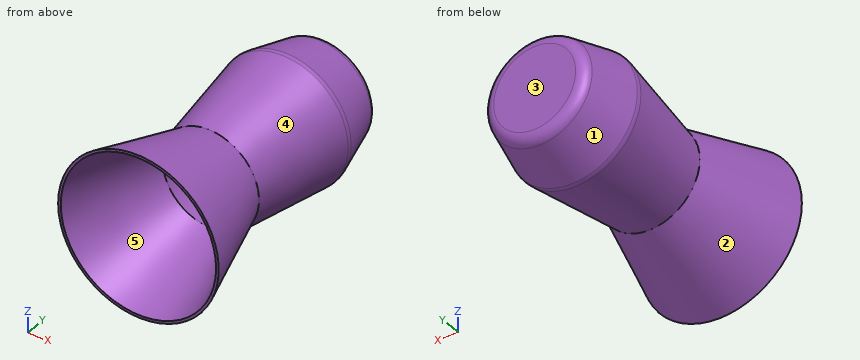
Autodesk Fusion 360 part; units mm, degrees
sketch "Esquisse1" plane through (0, 0, 0) normal (0, 0, 1) x (1, 0, 0)
  line L0 (0, 0) -> (-65, 0)
  line L1 (-65, 0) -> (-40, 80)
  line L2 (-40, 80) -> (-52.5, 165)
  line L3 (-52.5, 165) -> (-40, 210)
  line L4 (-40, 210) -> (0, 210)
  line L5 (0, 210) -> (0, 0)
  dimension "d1" = 65
  dimension "d3" = 45
  dimension "d4" = 85
  dimension "d5" = 80
  dimension "d6" = 40
  dimension "d7" = 52.5
  dimension "d8" = 40
revolve "Révolution1" add sketch "Esquisse1" angle 360 about axis through (0, 210, 0) along (0, -1, 0)
fillet "Congé1" radius 9 1 edges at (-48.9472, 165, 18.9848)
fillet "Congé2" radius 9 1 edges at (-37.2931, 210, 14.4646)
shell "Coque1" thickness 2 removed faces 1 at (20.2416, 0, -0.2148)
The model under review builds one solid part; all positions refer to its coordinate system, in mm. Face numbers are marked on the shaded views. A direction names the side the tool comes from. Round coordinates to 2 decimals unless told otherwise and drop trailing zeros. Order: outer loops, then holes, each group sorted by start corner. A loop starts at its lowest first (then second) coordinate and runs counter-clockwise, first axis right, second up. Notation, with made-up numbers: (78.25, 58) -> (124.25, 58) arc R20 ccw to (124.25, 88) -> close; hole circle Ø11 at (-5, 35.5). An arc over 180 degrees is marked (long way). One line per item, written item: value. Start each with the question number.
Q1. Clearance check with flat-ended pins moving along their axes: pin 1 Ø10 at (y, z) = (47, 43.5) entering from -X; pin 2 Ø8 at (y, z) = (167.5, -20.5) entering from -X; pin 3 Ø20 at (x, z) = (13, -3.5) entering from -Y. State where each tip first meets the part, or that it passes through.
Q2. Mouldability with a two-part tool opening along X and no side actions: class the marked faces 3, 4 and 5 as released by +X, released by -X, zero draft, split by the parting line, or undercut.
Q3. Machinability: for the marked faces 1 and 2, which of the approach directions +Z, -Z, +X, -X, +Y, -Y give a long, thin tool a straight path to every point of the face, cutting with its end or side? Answer none if there is none.
Q4. Take a section at A-A (y = 25). Write out the cut boundary in (x, z) (1 decimal), and give its area (3 significant figures).
Q5. Wall thickness on line 1 (Z direction, x = 10.5, y = 60); line 2 (X direction, y = 92, z = -15); line 3 (X direction, y = 52.5, z = 35): over which ranges is each line inside the solid? List them lowest first.
Reported:
1. pin 1: stops at x = -32.87
1. pin 2: stops at x = -49.41
1. pin 3: stops at y = 208
2. face 3: zero draft
2. face 4: split by the parting line
2. face 5: undercut
3. face 1: +Y
3. face 2: none
4. outline: circle Ø114.4 at (0, 0); hole circle Ø110.2 at (0, 0)
4. area: 739 mm2
5. line 1: z = -45.04 to -42.89, 42.89 to 45.04
5. line 2: x = -38.98 to -36.8, 36.8 to 38.98
5. line 3: x = -33.71 to -30.61, 30.61 to 33.71
